```python
from build123d import *

# Parameters (mm, degrees)
F1_DEPTH   = 4
F2_R       = 5
F3_R       = 5
F4_R       = 5
F5_R       = 5
F6_R       = 3
F7_SIZE2   = 2.5980762114
F7_SIZE    = 1.5
F7_2_SIZE2 = 2.5980762114
F7_2_SIZE  = 1.5
F7_3_SIZE2 = 2.5980762114
F7_3_SIZE  = 1.5
F7_4_SIZE2 = 2.5980762114
F7_4_SIZE  = 1.5
F7_5_SIZE2 = 2.5980762114
F7_5_SIZE  = 1.5
F7_6_SIZE2 = 2.5980762114
F7_6_SIZE  = 1.5


with BuildPart() as f1:
    # F0 (on Top) → F1 (new body)
    with BuildSketch(Plane.XY):
        with BuildLine():
            Line((84.0636147559, 40.0707364747), (-105.9363852441, 40.0707364747))
            Line((-105.9363852441, 40.0707364747), (-105.9363852441, 19.0707364747))
            Line((-105.9363852441, 19.0707364747), (-98.4363852441, 19.0707364747))
            ThreePointArc((-98.4363852441, 19.0707364747), (-95.9363852441, 21.5707364747), (-93.4363852441, 19.0707364747))
            Line((-93.4363852441, 19.0707364747), (-48.4363852441, 19.0707364747))
            ThreePointArc((-48.4363852441, 19.0707364747), (-45.9363852441, 21.5707364747), (-43.4363852441, 19.0707364747))
            Line((-43.4363852441, 19.0707364747), (21.5636147559, 19.0707364747))
            ThreePointArc((21.5636147559, 19.0707364747), (24.0636147559, 21.5707364747), (26.5636147559, 19.0707364747))
            Line((26.5636147559, 19.0707364747), (71.5636147559, 19.0707364747))
            ThreePointArc((71.5636147559, 19.0707364747), (74.0636147559, 21.5707364747), (76.5636147559, 19.0707364747))
            Line((76.5636147559, 19.0707364747), (84.0636147559, 19.0707364747))
            Line((84.0636147559, 19.0707364747), (84.0636147559, 40.0707364747))
        make_face()
        with BuildLine():
            Line((-98.4363852441, 19.0707364747), (-105.9363852441, 19.0707364747))
            Line((-105.9363852441, 19.0707364747), (-105.9363852441, -28.9292635253))
            Line((-105.9363852441, -28.9292635253), (-33.4363852441, -28.9292635253))
            ThreePointArc((-33.4363852441, -28.9292635253), (-30.9363852441, -26.4292635253), (-28.4363852441, -28.9292635253))
            Line((-28.4363852441, -28.9292635253), (6.5636147559, -28.9292635253))
            ThreePointArc((6.5636147559, -28.9292635253), (9.0636147559, -26.4292635253), (11.5636147559, -28.9292635253))
            Line((11.5636147559, -28.9292635253), (84.0636147559, -28.9292635253))
            Line((84.0636147559, -28.9292635253), (84.0636147559, 19.0707364747))
            Line((84.0636147559, 19.0707364747), (76.5636147559, 19.0707364747))
            ThreePointArc((76.5636147559, 19.0707364747), (74.0636147559, 16.5707364747), (71.5636147559, 19.0707364747))
            Line((71.5636147559, 19.0707364747), (26.5636147559, 19.0707364747))
            ThreePointArc((26.5636147559, 19.0707364747), (24.0636147559, 16.5707364747), (21.5636147559, 19.0707364747))
            Line((21.5636147559, 19.0707364747), (-43.4363852441, 19.0707364747))
            ThreePointArc((-43.4363852441, 19.0707364747), (-45.9363852441, 16.5707364747), (-48.4363852441, 19.0707364747))
            Line((-48.4363852441, 19.0707364747), (-93.4363852441, 19.0707364747))
            ThreePointArc((-93.4363852441, 19.0707364747), (-95.9363852441, 16.5707364747), (-98.4363852441, 19.0707364747))
        make_face()
        with BuildLine():
            Line((-33.4363852441, -28.9292635253), (-105.9363852441, -28.9292635253))
            Line((-105.9363852441, -28.9292635253), (-105.9363852441, -49.9292635253))
            Line((-105.9363852441, -49.9292635253), (84.0636147559, -49.9292635253))
            Line((84.0636147559, -49.9292635253), (84.0636147559, -28.9292635253))
            Line((84.0636147559, -28.9292635253), (11.5636147559, -28.9292635253))
            ThreePointArc((11.5636147559, -28.9292635253), (9.0636147559, -31.4292635253), (6.5636147559, -28.9292635253))
            Line((6.5636147559, -28.9292635253), (-28.4363852441, -28.9292635253))
            ThreePointArc((-28.4363852441, -28.9292635253), (-30.9363852441, -31.4292635253), (-33.4363852441, -28.9292635253))
        make_face()
    extrude(amount=F1_DEPTH)

    # F2
    f2_edges = [f1.edges().sort_by_distance(p)[0] for p in [
        (-105.936385, 40.070736, 2),
    ]]
    fillet(f2_edges, radius=F2_R)

    # F3
    f3_edges = [f1.edges().sort_by_distance(p)[0] for p in [
        (84.063615, 40.070736, 2),
    ]]
    fillet(f3_edges, radius=F3_R)

    # F4
    f4_edges = [f1.edges().sort_by_distance(p)[0] for p in [
        (84.063615, -49.929264, 2),
    ]]
    fillet(f4_edges, radius=F4_R)

    # F5
    f5_edges = [f1.edges().sort_by_distance(p)[0] for p in [
        (-105.936385, -49.929264, 2),
    ]]
    fillet(f5_edges, radius=F5_R)

    # F6
    f6_edges = [f1.edges().sort_by_distance(p)[0] for p in [
        (-10.936385, -49.929264, 4),
    ]]
    fillet(f6_edges, radius=F6_R)

    # F7
    f7_edges = [f1.edges().sort_by_distance(p)[0] for p in [
        (-98.436385, 19.070736, 4),
    ]]
    f7_side = f1.faces().sort_by_distance((-98.436385, 19.070736, 2))[0]
    chamfer(f7_edges, length=F7_SIZE, length2=F7_SIZE2, reference=f7_side)

    # F7#2
    f7_2_edges = [f1.edges().sort_by_distance(p)[0] for p in [
        (-48.436385, 19.070736, 4),
    ]]
    f7_2_side = f1.faces().sort_by_distance((-48.436385, 19.070736, 2))[0]
    chamfer(f7_2_edges, length=F7_2_SIZE, length2=F7_2_SIZE2, reference=f7_2_side)

    # F7#3
    f7_3_edges = [f1.edges().sort_by_distance(p)[0] for p in [
        (21.563615, 19.070736, 4),
    ]]
    f7_3_side = f1.faces().sort_by_distance((21.563615, 19.070736, 2))[0]
    chamfer(f7_3_edges, length=F7_3_SIZE, length2=F7_3_SIZE2, reference=f7_3_side)

    # F7#4
    f7_4_edges = [f1.edges().sort_by_distance(p)[0] for p in [
        (71.563615, 19.070736, 4),
    ]]
    f7_4_side = f1.faces().sort_by_distance((71.563615, 19.070736, 2))[0]
    chamfer(f7_4_edges, length=F7_4_SIZE, length2=F7_4_SIZE2, reference=f7_4_side)

    # F7#5
    f7_5_edges = [f1.edges().sort_by_distance(p)[0] for p in [
        (6.563615, -28.929264, 4),
    ]]
    f7_5_side = f1.faces().sort_by_distance((6.563615, -28.929264, 2))[0]
    chamfer(f7_5_edges, length=F7_5_SIZE, length2=F7_5_SIZE2, reference=f7_5_side)

    # F7#6
    f7_6_edges = [f1.edges().sort_by_distance(p)[0] for p in [
        (-33.436385, -28.929264, 4),
    ]]
    f7_6_side = f1.faces().sort_by_distance((-33.436385, -28.929264, 2))[0]
    chamfer(f7_6_edges, length=F7_6_SIZE, length2=F7_6_SIZE2, reference=f7_6_side)


solid = f1.part
```
Geometry check sheet. Reference: the model listing, model coordinates, mm. Coordinates: 2 decimals unless noted, no trailing zeros. One line per question, with ' | ' between items. Start each with the question number.
Item 1: Material ranges on L1, parallel to X at y = -28, z = 1.05; L2, parallel to X at y = 16, z = 3.75; L3, parallel to X at y = -41, z = 1.35, recorded low to high. Write a range as [from, to].
Item 2: Gauge pin test, flat ends, axial feed: pin 1 (4.5 mm diameter, centred on x = 24.06, y = 19.07, fed in from -Z); pin 2 (1.5 mm diameter, centred on y = -14, z = 2.5, fed in from +X); pin 3 (1 mm diameter, centred on x = 29, z = 2, fed in from -Y). Record the tip position at first contact, or that the pin passes through.
Item 3: Cross-section at A-A on z = 3.25. State how many separate pieces and enclosed holes the cut face has, then the cut area to 3 significant figures.
Findings:
1) L1: x = [-105.94, -33.26], [-28.62, 6.74], [11.38, 84.06] | L2: x = [-104.14, -99.45], [-92.42, -49.45], [-42.42, 20.55], [27.58, 70.55], [77.58, 82.26] | L3: x = [-105.92, 84.04]
2) pin 1: passes through | pin 2: stops at x = 83.97 | pin 3: stops at y = -49.89
3) separate pieces: 1 | enclosed holes: 6 | area: 16,200 mm²
